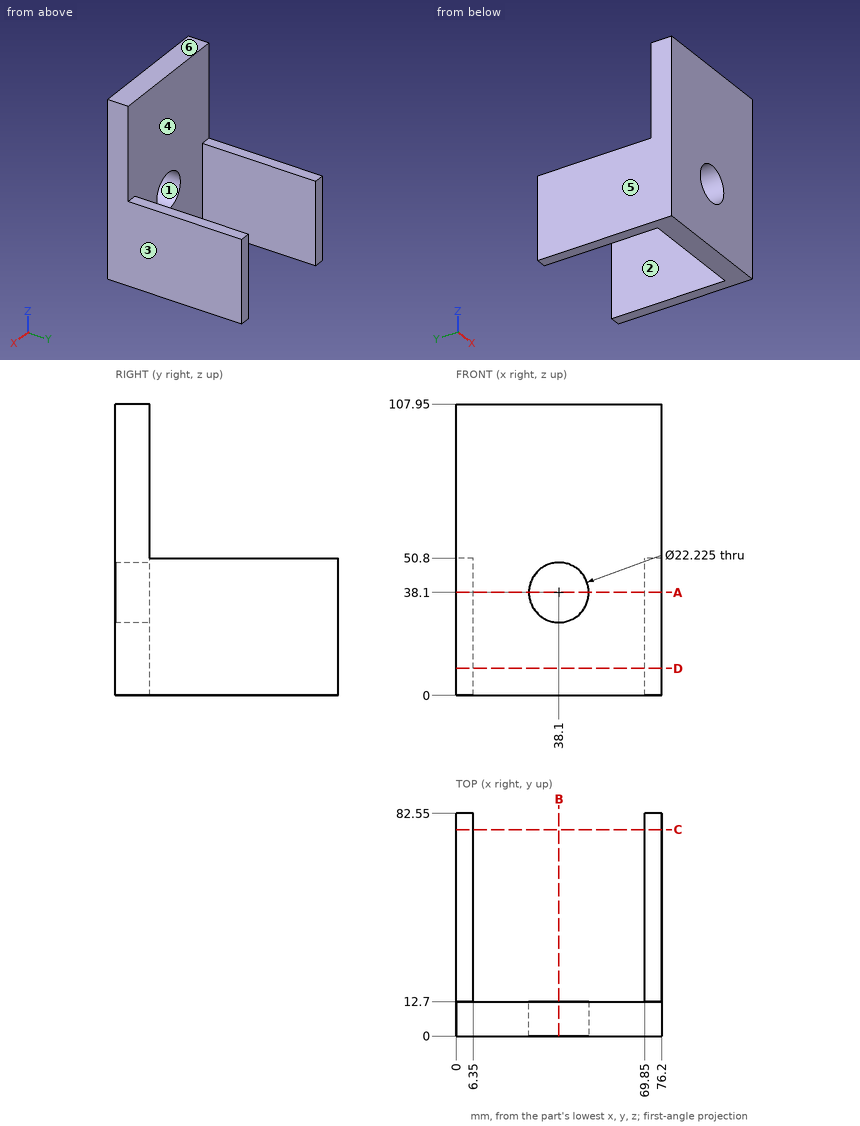
Check sheet for the drawn part. Datum: minimum x, y, z corner. Units: mm. A direction names the side the tool comes from. Give positions to 0.01 mm unless a question says otherwise; leave off trailing zeros. Order: outer loops, then holes, each group sorted by start corner. A loop starts at its lowest first (then second) coordinate and runs counter-clockwise, first axis right, second up. Notation, with made-up numbers: (72.25, 24.25) -> (126.25, 24.25) arc R15 cw to (126.25, 36.25) -> close; hole circle Ø1 at (85, 54.25). An arc over 180 degrees is marked (long way). Use a Markdown table: item, result.
1) Depth check by flat-ended pin: pin 1 Ø3 at (x, y) = (72.5, 46.5) entering from +Z; pin 2 Ø6 at (x, z) = (18, 20.5) entering from +Y; pin 3 Ø13.5 at (x, z) = (38.1, 38.1) entering from -Y. Enter the tip coordinate at first touch or a pass-through.
Results:
| item | result |
|---|---|
| pin 1 | z = 50.8 |
| pin 2 | y = 12.7 |
| pin 3 | through |
2) Section check A-A, the plane z = 38.1. Record the boundary of the cut face in (x, y).
Results:
| item | result |
|---|---|
| outline | (0, 0) -> (26.99, 0) -> (26.99, 12.7) -> (6.35, 12.7) -> (6.35, 82.55) -> (0, 82.55) -> close; (49.21, 0) -> (76.2, 0) -> (76.2, 82.55) -> (69.85, 82.55) -> (69.85, 12.7) -> (49.21, 12.7) -> close |
3) Tool access check on the marked faces 1 and 2. Record the directions out of +Z, -Z, +X, -X, +Y, -Y that give a thin tool (end or side, any length) a straight path to the whole face; none if there is none.
Results:
| item | result |
|---|---|
| face 1 | +Y, -Y |
| face 2 | +Z, -Z, +Y |
4) Section check D-D, the plane z = 10. Record the boundary of the cut face in (x, y).
Results:
| item | result |
|---|---|
| outline | (0, 0) -> (76.2, 0) -> (76.2, 82.55) -> (69.85, 82.55) -> (69.85, 12.7) -> (6.35, 12.7) -> (6.35, 82.55) -> (0, 82.55) -> close |
5) Mould release check, pull along X, two halves, no side actions. Record for the marked faces 3, 4, 5 and 6: pulls with the +X half, pulls with the -X half, needs draft (parallel to the pull), parting line crosses it, or undercut.
Results:
| item | result |
|---|---|
| face 3 | pulls with the +X half |
| face 4 | undercut |
| face 5 | pulls with the -X half |
| face 6 | needs draft |
6) Section check B-B, the plane x = 38.1. Record the boundary of the cut face in (y, z), then the cut area to 3 significant figures.
Results:
| item | result |
|---|---|
| outline | (0, 0) -> (12.7, 0) -> (12.7, 26.99) -> (0, 26.99) -> close; (0, 49.21) -> (12.7, 49.21) -> (12.7, 107.95) -> (0, 107.95) -> close |
| area | 1,090 mm² |
7) Section check C-C, the plane y = 76.5. Record the boundary of the cut face in (x, z).
Results:
| item | result |
|---|---|
| outline | (0, 0) -> (6.35, 0) -> (6.35, 50.8) -> (0, 50.8) -> close; (69.85, 0) -> (76.2, 0) -> (76.2, 50.8) -> (69.85, 50.8) -> close |
8) Material ranges on probe 1 along X at (y, z) = (39.5, 19); probe 2 along Z at (x, y) = (38.1, 6); probe 3 along X at (y, z) = (3, 38), recorded low to high.
Results:
| item | result |
|---|---|
| probe 1 | 0 to 6.35, 69.85 to 76.2 |
| probe 2 | 0 to 26.99, 49.21 to 107.95 |
| probe 3 | 0 to 26.99, 49.21 to 76.2 |
